Build history of the part. All positions in model axes, mm. A direction names the side the tool comes from. Round coordinates to 2 decimals unless told otherwise and drop trailing zeros. Write each loop counter-clockwise with the first axis right and the second up, starting at its lowest first coordinate (ties: lowest second). Pieces come first, ordered by that corner, then holes.
1) Wall check: probe 1 along X at (y, z) = (11, 6); probe 2 along X at (y, z) = (3.6, 3); probe 3 along X at (y, z) = (-13, -1.75). Give the ranges that are in metal, low to high.
2) Which spindle directions (+Z, -Z, +X, -X, +Y, -Y) get a long thin tool onto all of the face, cutting with end or side? Do faces 4 (the flat face through (12, -10.4, 0)), 5 (the flat face through (-9, 3, 0)), 6 (the flat face through (-1, 13, 0)), 7 (the flat face through (4, 13, -2)). Say none if no direction does.
3) Flat gauge pins, fed straight in: pin 1 (7 mm diameter, centred on y = 12, z = -1.5, fed in from +X); pin 2 (6.5 mm diameter, centred on x = 16, z = 0, fed in from +Y); pin 3 (3 mm diameter, centred on y = -7.5, z = 0, fed in from -X); pin 4 (4.5 mm diameter, centred on x = -16, z = 0, fed in from -Y). Where does each tip first touch, or does it go through?
4) Saw through at C-C (x = -1.5). Write the cut outline in (y, z).
5) Saw through at D-D (z = 4.5). Write the cut outline in (x, y).
6) Saw through at A-A (x = -16). Write the cut outline in (y, z), plus the area to 3 significant figures.
7) Saw through at B-B (y = 3.6). Write the cut outline in (x, z).
8) Pull direction X, two halves, no side cores. Call faces 1 (the cylindrical face through (-13.253, -13.485, 0.121)), 2 (the flat face through (21, -13, 0)), 3 (the flat face through (0, -7, 7)): +X half, -X half, draft (parallel to the pull), parting line (faces both ways), or undercut.
from build123d import *

# Parameters (mm, degrees)
EXTRUDE_1_DEPTH     = 7
SKETCH_2_R          = 2.75
CUT_EXTRUDE_1_DEPTH = 6
SKETCH_4_R          = 1.65
CUT_EXTRUDE_2_DEPTH = 8
SKETCH_5_R          = 2.1
CUT_EXTRUDE_3_DEPTH = 8
SKETCH_6_R          = 3.8
CUT_EXTRUDE_4_DEPTH = 5
CHAMFER_1_SIZE      = 0.25


with BuildPart() as part:
    # Эскиз1 → Бобышка-Вытянуть1 (new, symmetric)
    with BuildSketch(Plane.XY):
        with BuildLine():
            Line((-9, 16.4), (-1, 16.4))
            Line((-1, 16.4), (-1, 7.472983346))
            ThreePointArc((-1, 7.472983346), (0, -0.4), (1, 7.472983346))
            Line((1, 7.472983346), (1, 16.4))
            Line((1, 16.4), (9, 16.4))
            Line((9, 16.4), (9, -10.4))
            Line((9, -10.4), (21, -10.4))
            Line((21, -10.4), (21, -16.4))
            Line((21, -16.4), (-21, -16.4))
            Line((-21, -16.4), (-21, -10.4))
            Line((-21, -10.4), (-9, -10.4))
            Line((-9, -10.4), (-9, 16.4))
        make_face()
    extrude(amount=EXTRUDE_1_DEPTH, both=True)

    # Эскиз2 → Вырез-Вытянуть1 (cut)
    with BuildSketch(Plane(origin=(0, -10.4, 0), x_dir=(1, 0, 0), z_dir=(0, 1, 0))):
        with Locations(Location((-16, 0, 0), (0, 0, 180))):
            Circle(SKETCH_2_R)
        with Locations(Location((16, 0, 0), (0, 0, 180))):
            Circle(SKETCH_2_R)
    extrude(amount=-CUT_EXTRUDE_1_DEPTH, mode=Mode.SUBTRACT)

    # Эскиз4 → Вырез-Вытянуть2 (cut)
    with BuildSketch(Plane(origin=(-1, 0, 0), x_dir=(0, 0, -1), z_dir=(1, 0, 0))):
        with Locations((0, 10.936491673)):
            Circle(SKETCH_4_R)
    extrude(amount=-CUT_EXTRUDE_2_DEPTH, mode=Mode.SUBTRACT)

    # Эскиз5 → Вырез-Вытянуть3 (cut)
    with BuildSketch(Plane(origin=(9, 0, 0), x_dir=(0, 0, -1), z_dir=(1, 0, 0))):
        with Locations(Location((0, 10.936491673, 0), (0, 0, 90))):
            Circle(SKETCH_5_R)
    extrude(amount=-CUT_EXTRUDE_3_DEPTH, mode=Mode.SUBTRACT)

    # Эскиз6 → Вырез-Вытянуть4 (cut)
    with BuildSketch(Plane(origin=(9, 0, 0), x_dir=(0, 0, -1), z_dir=(1, 0, 0))):
        with Locations(Location((0, 10.936491673, 0), (0, 0, 90))):
            Circle(SKETCH_6_R)
    extrude(amount=-CUT_EXTRUDE_4_DEPTH, mode=Mode.SUBTRACT)

    # Фаска1
    chamfer_1_edges = [part.edges().sort_by_distance(p)[0] for p in [
        (-13.25, -10.4, 0),
        (18.75, -10.4, 0),
        (-9, 10.936491673, 1.65),
    ]]
    chamfer(chamfer_1_edges, length=CHAMFER_1_SIZE)


solid = part.part
Evaluation:
1. probe 1: x = -9 to -1, 1 to 9
1. probe 2: x = -9 to -4, 4 to 9
1. probe 3: x = -21 to -18.12, -13.88 to 13.88, 18.12 to 21
2. face 4: +Z, -Z, +X, +Y
2. face 5: +Z, -Z, -X, +Y
2. face 6: +Z, -Z, +Y
2. face 7: +X
3. pin 1: stops at x = 9
3. pin 2: stops at y = -10.4
3. pin 3: stops at x = -9
3. pin 4: passes through
4. outline: (-16.4, -7) - (-0.11, -7) - (-0.11, 7) - (-16.4, 7) - close; (7.31, -7) - (16.4, -7) - (16.4, 7) - (7.31, 7) - close; hole circle Ø3.3 at (10.94, 0)
5. outline: (-21, -16.4) - (21, -16.4) - (21, -10.4) - (9, -10.4) - (9, 16.4) - (1, 16.4) - (1, 7.47) arc R4 cw (long way) to (-1, 7.47) - (-1, 16.4) - (-9, 16.4) - (-9, -10.4) - (-21, -10.4) - close
6. outline: (-16.4, -7) - (-10.4, -7) - (-10.4, -3) - (-10.65, -2.75) - (-16.4, -2.75) - close; (-16.4, 2.75) - (-10.65, 2.75) - (-10.4, 3) - (-10.4, 7) - (-16.4, 7) - close
6. area: 50.9 mm2
7. outline: (-9, -7) - (-4, -7) - (-4, 7) - (-9, 7) - close; (4, -7) - (9, -7) - (9, 7) - (4, 7) - close
8. face 1: undercut
8. face 2: +X half
8. face 3: draft
